Input: part model. Units: mm. Frame: model coordinates. Face numbers are marked on the shaded views. Give positions to 0.01 mm unless a question says otherwise; leave off trailing zeros. Write each loop counter-clockwise with the first axis right and the second up, starting at its lowest first coordinate (ties: lowest second). Pieces come first, ordered by that corner, then holes. Notation, with made-up numbers: M 77,-32 L 88,-32 A9 ccw 88,-21 Z; hole C -35.75,-14.75 d5. An arc over 180 degrees is marked long. Use CSV: the item, a comma, the result in double quotes. Start each with the question number.
from build123d import *

# Parameters (mm, degrees)
F0_R     = 6
F0_R_2   = 4.25
F1_DEPTH = 10
F2_DEPTH = 8
F3_D     = 1.5


with BuildPart() as f1:
    # F0 (on Top) → F1 (new body)
    with BuildSketch(Plane.XY):
        with Locations((0, -0.5465864819)):
            Circle(F0_R)
        with Locations((0, -0.5465864819)):
            Circle(F0_R_2, mode=Mode.SUBTRACT)
        with Locations((0, -0.5465864819)):
            Circle(F0_R_2)
    extrude(amount=F1_DEPTH)

    # F0 (on Top) → F2 (cut)
    with BuildSketch(Plane.XY):
        with Locations((0, -0.5465864819)):
            Circle(F0_R_2)
    extrude(amount=F2_DEPTH, mode=Mode.SUBTRACT)

    # F3 (through all)
    with Locations(Plane(origin=(0, 0, 0), x_dir=(1, 0, 0), z_dir=(0, 0, -1))):
        with Locations((0, 0.5465864819)):
            Hole(F3_D / 2)


solid = f1.part
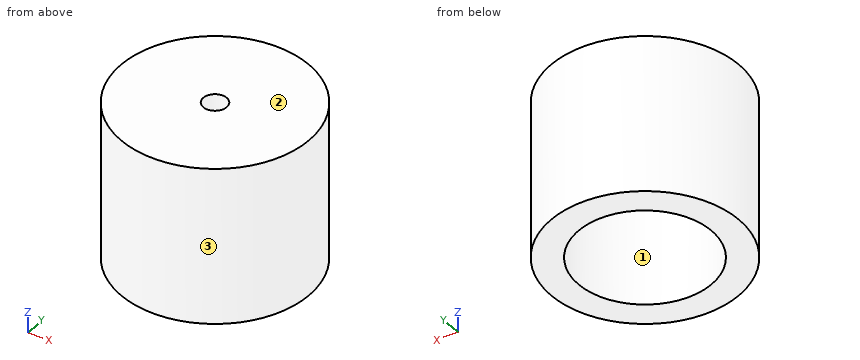
Q1. Section A-A, the plane x = 0. Return the cut outline in (y, z).
Q2. First-contact query: pin 1 Ø4 at (y, z) = (3.5, 4.5) entering from +X; pin 2 Ø6 at (x, z) = (4, 4) entering from -Y; pin 3 Ø4 at (y, z) = (-2.5, 4.5) entering from +X; pin 4 Ø5 at (y, z) = (-4.5, 5.5) entering from -X. Flat tips, straight axial feed; report the tip coordinate or a pass-through.
Q3. Section D-D, the plane x = 1.75. Return the cut outline in (y, z), and give its area (3 significant figures).
Q4. Material intervals for L1, parallel to Y at x = 0, z = 2; L2, parallel to Y at x = 0, z = 9; L3, parallel to Z at x = 2.5, y = -1.5, sorted ascending. Write a range as [from, to].
Q5. Section B-B, the plane y = 0. Return the cut outline in (x, z).
Q6. Pull-direction query (X, two-part tool) for the marked faces 1, 2 and 3; classes: released by +X, released by -X, zero draft, split by the parting line, or undercut.
Q7. Section C-C, the plane y = -1.75. Return the cut outline in (x, z).
Check result:
1,outline,"M -6.55,0 L -4.8,0 L -4.8,8 L -1.3,8 L -1.3,10 L -6.55,10 Z; M 0.2,8 L 3.7,8 L 3.7,0 L 5.45,0 L 5.45,10 L 0.2,10 Z"
2,pin 1,"stops at x = 5.64"
2,pin 2,"stops at y = -6.46"
2,pin 3,"stops at x = 6"
2,pin 4,"stops at x = -5.82"
3,outline,"M -6.29,0 L -4.42,0 L -4.42,8 L 3.33,8 L 3.33,0 L 5.19,0 L 5.19,10 L -6.29,10 Z"
3,area,"52.8 mm²"
4,L1,"y = [-6.55, -4.8], [3.7, 5.45]"
4,L2,"y = [-6.55, -1.3], [0.2, 5.45]"
4,L3,"z = [8, 10]"
5,outline,"M -5.98,0 L -4.21,0 L -4.21,8 L -0.51,8 L -0.51,10 L -5.98,10 Z; M 0.51,8 L 4.21,8 L 4.21,0 L 5.98,0 L 5.98,10 L 0.51,10 Z"
6,face 1,"undercut"
6,face 2,"zero draft"
6,face 3,"split by the parting line"
7,outline,"M -5.88,0 L -4.08,0 L -4.08,8 L 4.08,8 L 4.08,0 L 5.88,0 L 5.88,10 L -5.88,10 Z"
